The model under review builds one solid part; all positions refer to its coordinate system, in mm. Give positions to 0.01 mm unless a question says otherwise; leave off trailing zeros. Order: outer loops, then holes, each group sorted by start corner. A loop starts at its lowest first (then second) coordinate and runs counter-clockwise, first axis right, second up. Notation, with made-up numbers: (71.5, 70.25) -> (104.5, 70.25) arc R19 cw to (104.5, 105.25) -> close; hole circle Ø6 at (38, -25). An arc over 180 degrees is marked (long way). Use one line per item in the form item = value.
Autodesk Inventor part; units mm, degrees
ref_plane "Pracovní rovina1" through (1.5, 0, 0) normal (1, 0, 0) x (0, 0, -1)
ref_plane "Pracovní rovina2" through (-1.5, 0, 0) normal (-1, 0, 0) x (0, 0, 1)
ref_plane "YZ Plane" through (0, 0, 0) normal (1, 0, 0) x (0, 1, 0)
sketch "Náčrt1" plane through (0, 0, 0) normal (1, 0, 0) x (0, 1, 0)
  line L0 (19, 6.6) -> (31.312, 6.6)
  line L1 (31.312, -6.6) -> (19, -6.6)
  line L2 (19, -6.6) -> (19, 6.6)
  line L3 (24.8085, 20.2123) -> (16.7938, 12.1976)
  line L4 (16.7938, 12.1976) -> (12.1976, 16.7938)
  line L5 (12.1976, 16.7938) -> (20.2123, 24.8085)
  line L6 (0, 0) -> (14.4957, 14.4957)
  line L7 (6.6, 19) -> (-6.6, 19)
  line L8 (6.6, 31.312) -> (6.6, 19)
  line L9 (-6.6, 19) -> (-6.6, 31.312)
  line L10 (-20.2123, 24.8085) -> (-12.1976, 16.7938)
  line L11 (-12.1976, 16.7938) -> (-16.7938, 12.1976)
  line L12 (-16.7938, 12.1976) -> (-24.8085, 20.2123)
  line L13 (-19, 6.6) -> (-19, -6.6)
  line L14 (-31.312, 6.6) -> (-19, 6.6)
  line L15 (-19, -6.6) -> (-31.312, -6.6)
  line L16 (-24.8085, -20.2123) -> (-16.7938, -12.1976)
  line L17 (-16.7938, -12.1976) -> (-12.1976, -16.7938)
  line L18 (-12.1976, -16.7938) -> (-20.2123, -24.8085)
  line L19 (-6.6, -19) -> (6.6, -19)
  line L20 (-6.6, -31.312) -> (-6.6, -19)
  line L21 (6.6, -19) -> (6.6, -31.312)
  line L22 (20.2123, -24.8085) -> (12.1976, -16.7938)
  line L23 (12.1976, -16.7938) -> (16.7938, -12.1976)
  line L24 (16.7938, -12.1976) -> (24.8085, -20.2123)
  arc A0 (24.8085, -20.2123) -> (31.312, -6.6) centre (0, 0) ccw
  arc A1 (6.6, -31.312) -> (20.2123, -24.8085) centre (0, 0) ccw
  arc A2 (-20.2123, -24.8085) -> (-6.6, -31.312) centre (0, 0) ccw
  arc A3 (-31.312, -6.6) -> (-24.8085, -20.2123) centre (0, 0) ccw
  arc A4 (-24.8085, 20.2123) -> (-31.312, 6.6) centre (0, 0) ccw
  arc A5 (-6.6, 31.312) -> (-20.2123, 24.8085) centre (0, 0) ccw
  arc A6 (31.312, 6.6) -> (24.8085, 20.2123) centre (0, 0) ccw
  arc A7 (20.2123, 24.8085) -> (6.6, 31.312) centre (0, 0) ccw
  line L25 (16.205, 20.8011) -> (20.8011, 16.205)
  line L26 (14.9675, 23.4528) -> (13.5533, 22.0386)
  line L27 (13.5533, 22.0386) -> (22.0386, 13.5533)
  line L28 (22.0386, 13.5533) -> (23.4528, 14.9675)
  line L29 (23.4528, 14.9675) -> (14.9675, 23.4528)
  line L30 (-13.5533, 22.0386) -> (-14.9675, 23.4528)
  line L31 (-22.0386, 13.5533) -> (-13.5533, 22.0386)
  line L32 (-14.9675, 23.4528) -> (-23.4528, 14.9675)
  line L33 (-23.4528, 14.9675) -> (-22.0386, 13.5533)
  line L34 (-22.0386, -13.5533) -> (-23.4528, -14.9675)
  line L35 (-13.5533, -22.0386) -> (-22.0386, -13.5533)
  line L36 (-23.4528, -14.9675) -> (-14.9675, -23.4528)
  line L37 (-14.9675, -23.4528) -> (-13.5533, -22.0386)
  line L38 (13.5533, -22.0386) -> (14.9675, -23.4528)
  line L39 (22.0386, -13.5533) -> (13.5533, -22.0386)
  line L40 (14.9675, -23.4528) -> (23.4528, -14.9675)
  line L41 (23.4528, -14.9675) -> (22.0386, -13.5533)
  point P0 (-14.4957, 14.4957)
  point P1 (-14.4957, -14.4957)
  point P2 (14.4957, -14.4957)
  dimension "d1" = 6.6
  dimension "d2" = 6.6
  dimension "d4" = 6.5
  dimension "d5" = 3.25
  dimension "d6" = 20.5
  dimension "d7" = 45
  dimension "d10" = 360
  dimension "d12" = 2
  dimension "d13" = 12
  dimension "d14" = 1
  dimension "d15" = 2.75
  dimension "d18" = 360
extrude "Vysunutí1" add sketch "Náčrt1" along normal mid plane 3 contours L2 L1 A0 L24 L40 L41 L39 L23 L22 L38 A1 L21 L19 L20 A2 L18 L36 L37 L35 L17 L16 L34 A3 L15 L13 L14 A4 L12 L32 L33 L31 L11 L10 L30 A5 L9 L7 L8 A7 L5 L29 L26 L27 L4 L3 L28 A6 L0 | L29 L28 L27 L3 | L5 L27 L26 L29 | L24 L39 L41 L40 | L40 L38 L39 L22 | L32 L30 L31 L10 | L12 L31 L33 L32 | L18 L35 L37 L36 | L36 L34 L35 L16
ref_plane "Pracovní rovina1" through (1.5, 0, 0) normal (1, 0, 0) x (0, 0, -1)
sketch "Náčrt3" plane through (1.5, 0, 0) normal (1, 0, 0) x (0, 0, -1)
  line L0 (-11.5, 7) -> (-11.5, -7)
  line L1 (11.5, -7) -> (11.5, 7)
  arc A0 (5, 7) -> (-5, 7) centre (0, 7) ccw
  arc A1 (-5, -7) -> (5, -7) centre (0, -7) ccw
  line L2 (-11.5, -7) -> (-5, -7)
  line L3 (5, -7) -> (11.5, -7)
  line L4 (11.5, 7) -> (5, 7)
  line L5 (-5, 7) -> (-11.5, 7)
  point P0 (0, 0)
  dimension "d34" = 23
  dimension "d35" = 14
  dimension "d37" = 11.5
  dimension "d38" = 10
  dimension "d39" = 10
extrude "Vysunutí3" cut sketch "Náčrt3" against normal blind 4
ref_plane "Pracovní rovina2" through (-1.5, 0, 0) normal (-1, 0, 0) x (0, 0, 1)
sketch "Náčrt4" plane through (-1.5, 0, 0) normal (-1, 0, 0) x (0, 0, 1)
  line L0 (-11.5, 7) -> (-5, 7)
  arc A0 (5, 7) -> (-5, 7) centre (0, 7) ccw
  line L1 (5, 7) -> (11.5, 7)
  line L2 (11.5, 7) -> (11.5, -7)
  line L3 (11.5, -7) -> (5, -7)
  arc A1 (-5, -7) -> (5, -7) centre (0, -7) ccw
  line L4 (-5, -7) -> (-11.5, -7)
  line L5 (-11.5, -7) -> (-11.5, 7)
  line L6 (6.6, 31.312) -> (6.6, 19)
  line L7 (6.6, 19) -> (-6.6, 19)
  line L8 (-6.6, 19) -> (-6.6, 31.312)
  arc A2 (-6.6, 31.312) -> (-20.2123, 24.8085) centre (0, 0) ccw
  line L9 (-20.2123, 24.8085) -> (-12.1976, 16.7938)
  line L10 (-12.1976, 16.7938) -> (-16.7938, 12.1976)
  line L11 (-16.7938, 12.1976) -> (-24.8085, 20.2123)
  arc A3 (-24.8085, 20.2123) -> (-31.312, 6.6) centre (0, 0) ccw
  line L12 (-31.312, 6.6) -> (-19, 6.6)
  line L13 (-19, 6.6) -> (-19, -6.6)
  line L14 (-19, -6.6) -> (-31.312, -6.6)
  arc A4 (-31.312, -6.6) -> (-24.8085, -20.2123) centre (0, 0) ccw
  line L15 (-24.8085, -20.2123) -> (-16.7938, -12.1976)
  line L16 (-16.7938, -12.1976) -> (-12.1976, -16.7938)
  line L17 (-12.1976, -16.7938) -> (-20.2123, -24.8085)
  arc A5 (-20.2123, -24.8085) -> (-6.6, -31.312) centre (0, 0) ccw
  line L18 (-6.6, -31.312) -> (-6.6, -19)
  line L19 (-6.6, -19) -> (6.6, -19)
  line L20 (6.6, -19) -> (6.6, -31.312)
  arc A6 (6.6, -31.312) -> (20.2123, -24.8085) centre (0, 0) ccw
  line L21 (20.2123, -24.8085) -> (12.1976, -16.7938)
  line L22 (12.1976, -16.7938) -> (16.7938, -12.1976)
  line L23 (16.7938, -12.1976) -> (24.8085, -20.2123)
  arc A7 (24.8085, -20.2123) -> (31.312, -6.6) centre (0, 0) ccw
  line L24 (31.312, -6.6) -> (19, -6.6)
  line L25 (19, -6.6) -> (19, 6.6)
  line L26 (19, 6.6) -> (31.312, 6.6)
  arc A8 (31.312, 6.6) -> (24.8085, 20.2123) centre (0, 0) ccw
  line L27 (24.8085, 20.2123) -> (16.7938, 12.1976)
  line L28 (16.7938, 12.1976) -> (12.1976, 16.7938)
  line L29 (12.1976, 16.7938) -> (20.2123, 24.8085)
  arc A9 (20.2123, 24.8085) -> (6.6, 31.312) centre (0, 0) ccw
  line L30 (16.7938, 12.1976) -> (12.1976, 16.7938)
  line L31 (-16.7938, -12.1976) -> (-12.1976, -16.7938)
sketch "Náčrt5" plane through (-1.5, 0, 0) normal (-1, 0, 0) x (0, 0, 1)
  circle A0 centre (10, -10) radius 1.55
  circle A1 centre (10, 10) radius 1.55
  circle A2 centre (-10, 10) radius 1.55
  circle A3 centre (-10, -10) radius 1.55
  point P0 (0, 0)
  dimension "d45" = 360
  dimension "d47" = 10
  dimension "d48" = 10
  dimension "d49" = 3.1
extrude "Vysunutí4" cut sketch "Náčrt5" against normal blind 4
sketch "Náčrt6" plane through (1.5, 0, 0) normal (1, 0, 0) x (0, 0, -1)
  circle A0 centre (10, 25) radius 1.55
  circle A1 centre (-10, 25) radius 1.55
  circle A2 centre (-25, 10) radius 1.55
  circle A3 centre (-25, -10) radius 1.55
  circle A4 centre (-10, -25) radius 1.55
  circle A5 centre (10, -25) radius 1.55
  circle A6 centre (25, -10) radius 1.55
  circle A7 centre (25, 10) radius 1.55
  point P0 (0, 0)
  dimension "d52" = 3.1
  dimension "d53" = 3.1
  dimension "d54" = 25
  dimension "d55" = 25
  dimension "d56" = 10
  dimension "d57" = 10
  dimension "d60" = 360
sketch "Sketch7" plane through (-1.5, 16.7938, 12.1976) normal (0, -0.7071, 0.7071) x (1, 0, 0)
  circle A0 centre (2.9795, 4.3345) radius 1
  line L0 (0, 11.3345) -> (3, 11.3345)
  point P0 (1.5, -20.5)
  dimension "d64" = 2
  dimension "d65" = 7
extrude "Extrusion6" cut sketch "Sketch7" against normal blind 3 and the other way blind 9
pattern_circular "Circular Pattern1" count 4 over 360 about axis through (0, 0, 0) along (1, 0, 0) of "Extrusion6"
sketch "Sketch8" plane through (-1.5, 0, 0) normal (-1, 0, 0) x (0, 0, 1)
  circle A0 centre (10, 25) radius 1.55
  circle A1 centre (-10, 25) radius 1.55
  circle A2 centre (-25, 10) radius 1.55
  circle A3 centre (-25, -10) radius 1.55
  circle A4 centre (-10, -25) radius 1.55
  circle A5 centre (10, -25) radius 1.55
  circle A6 centre (25, -10) radius 1.55
  circle A7 centre (25, 10) radius 1.55
  point P0 (0, 0)
  dimension "d73" = 3.1
  dimension "d74" = 3.1
  dimension "d75" = 25
  dimension "d76" = 25
  dimension "d77" = 10
  dimension "d78" = 10
  dimension "d79" = 360
hole "Hole1" at (-1.5, -25, 10) at (-1.5, -10, 25) at (-1.5, 10, 25) at (-1.5, 25, 10) at (-1.5, 25, -10) at (-1.5, 10, -25) at (-1.5, -10, -25) at (-1.5, -25, -10) direction (1, 0, 0) diameter 3.1 end through all countersink diameter 6 countersink angle 90
equation "\"d5\" = 0.5 * d4"
equation "\"d14\" = 0.5 * d12"
equation "\"d15\" = -0.5 * d4 + 0.5 * d13"
equation "\"d39\" = d38"
equation "\"d36\" = 0.5 * d35"
properties part number "deska"
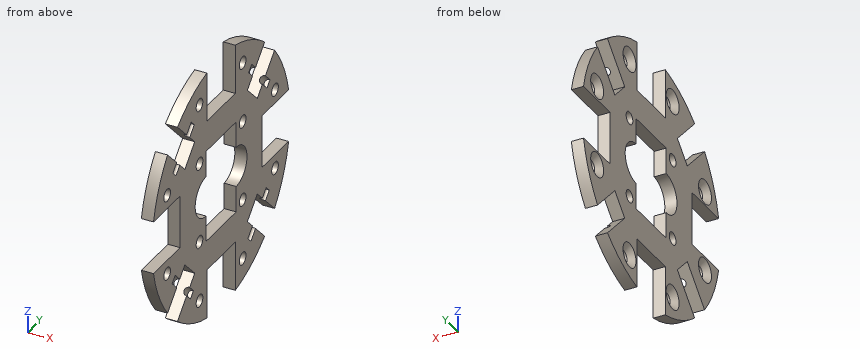
1. For L1, parallel to Y at x = -0.8, z = -10; L2, parallel to Y at x = 0.5, z = 10; L3, parallel to Z at x = 1.2, y = -13, list the stretches that pass through material, from the lowest coordinate up.
Values:
L1 = -30.4 to -27.3, -22.7 to -11.55, -8.45 to -7, 7 to 8.45, 11.55 to 22.7, 27.3 to 30.4
L2 = -30.4 to -26.55, -23.45 to -11.55, -8.45 to -7, 7 to 8.45, 11.55 to 23.45, 26.55 to 30.4
L3 = -29.24 to -21.13, -20.76 to -17.6, -15.99 to 15.99, 17.6 to 20.76, 21.84 to 29.24
2. For pin 1 Ø0.9 at (x, z) = (-0.5, -8) entering from +Y; pin 2 Ø1 at (x, y) = (1, -8) entering from +Z; pin 3 Ø3 at (y, z) = (25, 10) entering from -X; pin 4 Ø8 at (y, z) = (13.5, -21.5) entering from +X, all flat-tipped, find the tip position at first contact; note any pin that passes through.
Values:
pin_1 = 31.1
pin_2 = 31.11
pin_3 = through
pin_4 = 1.5
3. Add section B-B on z = 0. Give the boundary of the cut face in (x, y).
Values:
outline = (-1.5, -19) -> (1.5, -19) -> (1.5, -12) -> (-1.5, -12) -> close; (-1.5, 12) -> (1.5, 12) -> (1.5, 19) -> (-1.5, 19) -> close
4. Add section D-D on y = 10. Give the boundary of the cut face in (x, z).
Values:
outline = (-1.5, -30.4) -> (1.5, -30.4) -> (1.5, -26.55) -> (-0.05, -26.55) -> (-1.5, -28) -> close; (-1.5, -22) -> (-0.05, -23.45) -> (1.5, -23.45) -> (1.5, -11.55) -> (-1.5, -11.55) -> close; (-1.5, -8.45) -> (1.5, -8.45) -> (1.5, -4) -> (-1.5, -4) -> close; (-1.5, 4) -> (1.5, 4) -> (1.5, 8.45) -> (-1.5, 8.45) -> close; (-1.5, 11.55) -> (1.5, 11.55) -> (1.5, 23.45) -> (-0.05, 23.45) -> (-1.5, 22) -> close; (-1.5, 28) -> (-0.05, 26.55) -> (1.5, 26.55) -> (1.5, 30.4) -> (-1.5, 30.4) -> close
5. Add section A-A on y = -4. Give the boundary of the cut face in (x, z), then the cut area to 3 significant figures.
Values:
outline = (-1.5, -19) -> (1.5, -19) -> (1.5, -11.5) -> (-1.5, -11.5) -> close; (-1.5, 11.5) -> (1.5, 11.5) -> (1.5, 19) -> (-1.5, 19) -> close
area = 45.0 mm^2
6. Add section C-C on z = 10. Give the boundary of the cut face in (x, y).
Values:
outline = (-1.5, -30.4) -> (1.5, -30.4) -> (1.5, -26.55) -> (-0.05, -26.55) -> (-1.5, -28) -> close; (-1.5, -22) -> (-0.05, -23.45) -> (1.5, -23.45) -> (1.5, -11.55) -> (-1.5, -11.55) -> close; (-1.5, -8.45) -> (1.5, -8.45) -> (1.5, -7) -> (-1.5, -7) -> close; (-1.5, 7) -> (1.5, 7) -> (1.5, 8.45) -> (-1.5, 8.45) -> close; (-1.5, 11.55) -> (1.5, 11.55) -> (1.5, 23.45) -> (-0.05, 23.45) -> (-1.5, 22) -> close; (-1.5, 28) -> (-0.05, 26.55) -> (1.5, 26.55) -> (1.5, 30.4) -> (-1.5, 30.4) -> close
